from build123d import *

# Parameters (mm, degrees)
SKETCH1_W                  = 17.5
SKETCH1_H                  = 10
BASE_FLANGE1_DEPTH         = 2
F_4_CLEARANCE_HOLE1_D      = 3.2639
F_4_CLEARANCE_HOLE1_DEPTH  = 2
F_4_CLEARANCE_HOLE1_TIP    = 0.980574487
EDGE_FLANGE2_DEPTH         = 17.5
EDGE_FLANGE3_DEPTH         = 17.5
F_10_CLEARANCE_HOLE1_D     = 5.1054
F_10_CLEARANCE_HOLE1_DEPTH = 7.6
F_10_CLEARANCE_HOLE1_TIP   = 1.533816902


# Sheet-metal steps are written as plain solids
with BuildPart() as part:
    # Sketch1 → Base-Flange1 (new body)
    with BuildSketch(Plane(origin=(0, 0, 0), x_dir=(1, 0, 0), z_dir=(0, 1, 0))):
        with Locations((-14.536713287, 16.32983683)):
            Rectangle(SKETCH1_W, SKETCH1_H)
    extrude(amount=-BASE_FLANGE1_DEPTH)

    # #4 Clearance Hole1
    with Locations(Plane.XZ.offset(2)):
        with Locations((-9.786713287, -16.32983683), (-19.286713287, -16.32983683)):
            Hole(F_4_CLEARANCE_HOLE1_D / 2, depth=F_4_CLEARANCE_HOLE1_DEPTH)
            with Locations((0, 0, -(F_4_CLEARANCE_HOLE1_DEPTH + F_4_CLEARANCE_HOLE1_TIP / 2))):  # 118° drill point
                Cone(0, F_4_CLEARANCE_HOLE1_D / 2, F_4_CLEARANCE_HOLE1_TIP, mode=Mode.SUBTRACT)

    # Edge-Flange2 section (across the edge) → Edge-Flange2 (add)
    with BuildSketch(Plane(origin=(-23.286713287, 0, -10.59323683), x_dir=(0, 0, -1), z_dir=(1, 0, 0))):
        with BuildLine():
            Line((-2, 0.7366), (-2, 27.8))
            Line((-2, 27.8), (0, 27.8))
            Line((0, 27.8), (0, 0.7366))
            ThreePointArc((0, 0.7366), (0.215745145, 0.215745145), (0.7366, 0))
            Line((0.7366, 0), (0.7366, -2))
            ThreePointArc((0.7366, -2), (-1.198468417, -1.198468417), (-2, 0.7366))
        make_face()
    extrude(amount=EDGE_FLANGE2_DEPTH)

    # Edge-Flange3 section (across the edge) → Edge-Flange3 (add)
    with BuildSketch(Plane(origin=(-5.786713287, 28.5366, -8.59323683), x_dir=(0, -1, 0), z_dir=(-1, 0, 0))):
        with BuildLine():
            Line((-2, 0.7366), (-2, 20))
            Line((-2, 20), (0, 20))
            Line((0, 20), (0, 0.7366))
            ThreePointArc((0, 0.7366), (0.215745145, 0.215745145), (0.7366, 0))
            Line((0.7366, 0), (0.7366, -2))
            ThreePointArc((0.7366, -2), (-1.198468417, -1.198468417), (-2, 0.7366))
        make_face()
    extrude(amount=EDGE_FLANGE3_DEPTH)

    # #10 Clearance Hole1
    with Locations(Plane(origin=(0, 28.5366, 0), x_dir=(-1, 0, 0), z_dir=(0, -1, 0))):
        with Locations((14.536713287, 0.85663683)):
            Hole(F_10_CLEARANCE_HOLE1_D / 2, depth=F_10_CLEARANCE_HOLE1_DEPTH)
            with Locations((0, 0, -(F_10_CLEARANCE_HOLE1_DEPTH + F_10_CLEARANCE_HOLE1_TIP / 2))):  # 118° drill point
                Cone(0, F_10_CLEARANCE_HOLE1_D / 2, F_10_CLEARANCE_HOLE1_TIP, mode=Mode.SUBTRACT)


solid = part.part
Build history of the part. All positions in model axes, mm. A direction names the side the tool comes from. Give positions to 0.01 mm unless a question says otherwise; leave off trailing zeros. Write each loop counter-clockwise with the first axis right and the second up, starting at its lowest first coordinate (ties: lowest second). Pieces come first, ordered by that corner, then holes. Notation, with made-up numbers: (73, -0.5) - (121, -0.5) arc R18 cw to (121, 32.5) - close; hole circle Ø4 at (53, 17.5). An arc over 180 degrees is marked (long way). Use one line per item in the form item = value. Start each with the question number.
1. Probe line 1 (Y direction, x = -10.5, z = -14); line 2 (Y direction, x = -12.5, z = 2); line 3 (Z direction, x = -18.25, y = 22.5). List the from-to ranges inside material, lowest first. Write a range as [from, to].
2. Band-saw the part on D-D on x = -10.25. Write the cut outline in (y, z), plus the area to 3 significant figures.
3. Two-plate mould, pull along Z, no slides. Class faces 1 (the face through (-15, 0, -16)), 2 (the face through (-9.433, -0.986, -17.923)), 3 (the face through (-17.087, 29.551, -0.969)), 4 (the face through (-14.414, 29.714, -9.813)): released by +Z, released by -Z, zero draft, split by the parting line, or undercut.
4. Band-saw the part on C-C on y = 4. Write the cut outline in (x, z).
5. 3-axis set-ups, long thin cutter, end or side, ignore diameter. For faces 5 (the face through (-12, 30.537, 2)), 6 (the face through (-15, 14, -10.593)), 7 (the face through (-15, 14, -8.593)): which of +Z, -Z, +X, -X, +Y, -Y reach the whole face in a straight line?
6. Band-saw the part on A-A on z = -2. Write the cut outline in (x, y), plus the area to 3 significant figures.
7. Drop flat-ended pins along their axis: pin 1 Ø2 at (x, y) = (-11.5, 2.5) entering from +Z; pin 2 Ø9 at (x, z) = (-15, -1.5) entering from -Y; pin 3 Ø3 at (x, z) = (-13.5, -17) entering from +Y; pin 4 Ø4 at (x, z) = (-14.54, -0.86) entering from -Y. Give the stop position or say it passes through.
8. Band-saw the part on B-B on x = -19.5. Write the cut outline in (y, z), plus the area to 3 significant figures.
Conclusion:
q1.line_1 = [-2, 0]
q1.line_2 = [28.54, 30.54]
q1.line_3 = [-10.59, -8.59]
q2.outline = (-2, -21.33) - (0, -21.33) - (0, -17.89) - (-2, -17.89) - close; (-2, -14.77) - (0, -14.77) - (0, -11.33) arc R0.74 cw to (0.74, -10.59) - (27.8, -10.59) arc R2.74 ccw to (30.54, -7.86) - (30.54, 11.41) - (28.54, 11.41) - (28.54, -7.86) arc R0.74 cw to (27.8, -8.59) - (0.74, -8.59) arc R2.74 ccw to (-2, -11.33) - close
q2.area = 117 mm²
q3.face_1 = zero draft
q3.face_2 = undercut
q3.face_3 = undercut
q3.face_4 = released by -Z
q4.outline = (-23.29, -10.59) - (-5.79, -10.59) - (-5.79, -8.59) - (-23.29, -8.59) - close
q5.face_5 = +Z, -Z, +X, -X, +Y
q5.face_6 = -Z, +X, -X, +Y
q5.face_7 = +Z, +X, -X, -Y
q6.outline = (-23.29, 28.54) - (-16.82, 28.54) - (-16.82, 30.54) - (-23.29, 30.54) - close; (-12.25, 28.54) - (-5.79, 28.54) - (-5.79, 30.54) - (-12.25, 30.54) - close
q6.area = 25.9 mm²
q7.pin_1 = -8.59
q7.pin_2 = 28.54
q7.pin_3 = 0
q7.pin_4 = through
q8.outline = (-2, -21.33) - (0, -21.33) - (0, -17.95) - (-2, -17.95) - close; (-2, -14.71) - (0, -14.71) - (0, -11.33) arc R0.74 cw to (0.74, -10.59) - (27.8, -10.59) arc R2.74 ccw to (30.54, -7.86) - (30.54, 11.41) - (28.54, 11.41) - (28.54, -7.86) arc R0.74 cw to (27.8, -8.59) - (0.74, -8.59) arc R2.74 ccw to (-2, -11.33) - close
q8.area = 117 mm²
